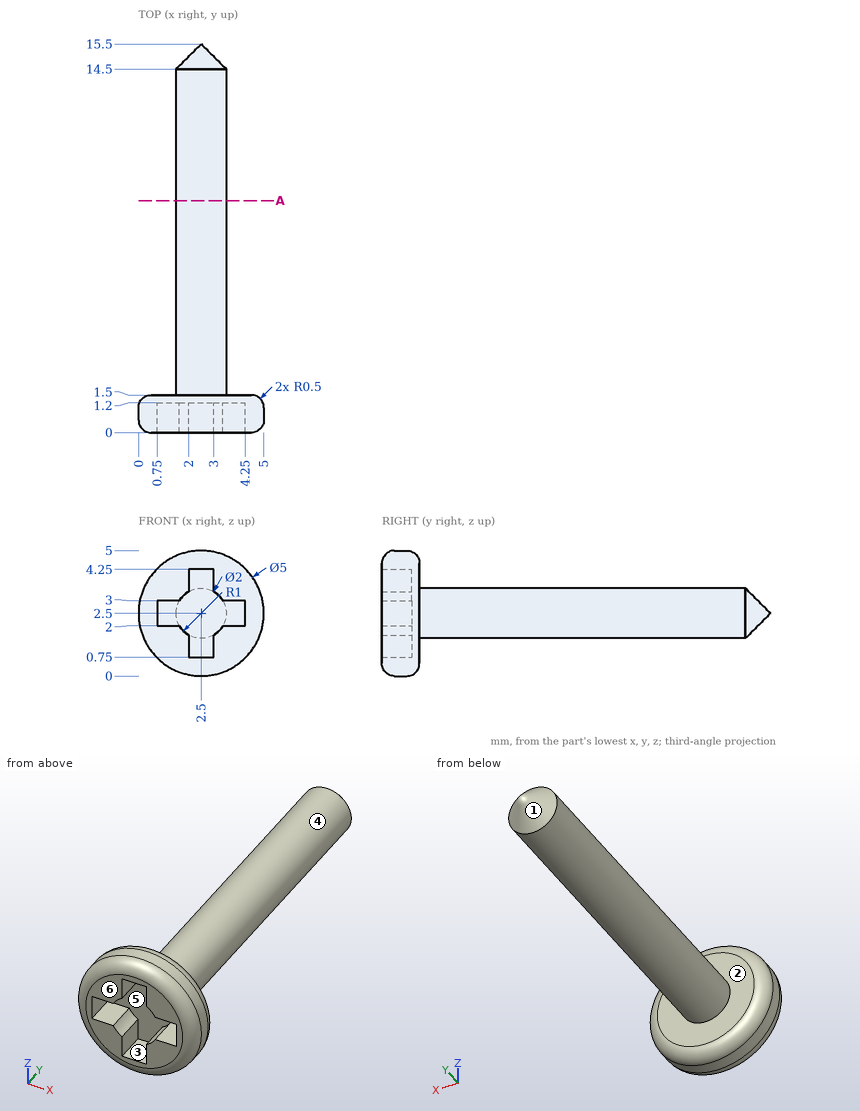
Answer from the drawing. Dimensions are ordinates in mm from the lowest x, y and z of the part. A direction names the side the tool comes from. Round coordinates to 2 decimals unless told otherwise and drop trailing zeros. Write each loop counter-clockwise with the first axis right and the second up, starting at its lowest first coordinate (ties: lowest second). Pieces come first, ordered by that corner, then holes. Notation, with made-up numbers: (-33, -16) - (-28, -16) arc R10 cw to (-28, -6) - close; hole circle Ø10 at (-26, 46.5). An arc over 180 degrees is marked (long way). Use a Markdown table: item, result.
(1) Each of these flat-tipped pins is pushed along its axis until it touches: pin 1 Ø2 at (x, z) = (4, 4.5) entering from +Y; pin 2 Ø1 at (x, y) = (4, 1) entering from +Z; pin 3 Ø1.5 at (x, y) = (4.5, 12.5) entering from +Z; pin 4 Ø1 at (y, z) = (1, 4) entering from +X. Where does it stop, or does it pass through?
Reported:
| item | result |
|---|---|
| pin 1 | y = 1.5 |
| pin 2 | z = 4.79 |
| pin 3 | through |
| pin 4 | x = 4.79 |
(2) The part is cut by section A-A (y = 9.25). Write down the section's boundary in (x, z).
Reported:
| item | result |
|---|---|
| outline | circle Ø2 at (2.5, 2.5) |
(3) The mould has two halves that part along X. Classify the marked faces 1, 2 and 3: released by +X, released by -X, zero draft, split by the parting line, or undercut.
Reported:
| item | result |
|---|---|
| face 1 | split by the parting line |
| face 2 | zero draft |
| face 3 | undercut |
(4) Which of the six approach directions +Z, -Z, +X, -X, +Y, -Y give full straight-line access (tool end or side, diameter ignored) to the marked faces 4, 5 and 6?
Reported:
| item | result |
|---|---|
| face 4 | +Y |
| face 5 | -Y |
| face 6 | +Z, -Z, +X, -X, -Y |
(5) Straight lines are drawn through the part: line 1 along Y through (x, z) = (2.55, 4.3); line 2 along Z through (x, y) = (3.4, 6.75); line 3 along Y through (x, z) = (2.55, 3.15). For each, find the intervals that lie inside material, in ascending order. Write a range as [from, to].
Reported:
| item | result |
|---|---|
| line 1 | [0, 1.5] |
| line 2 | [2.06, 2.94] |
| line 3 | [1.2, 14.85] |
